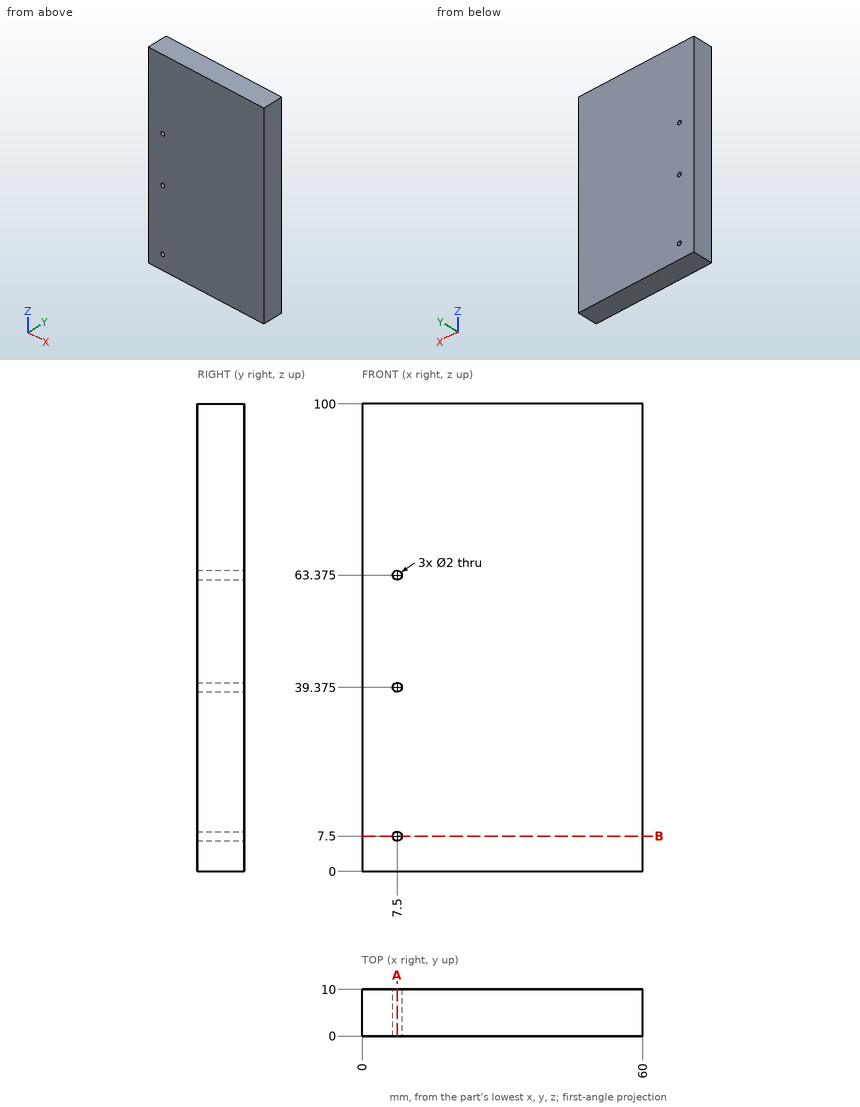
Geometry: see drawing. Coordinates: mm, zero at the bounding-box minimum. Coordinates: 2 decimals unless noted, no trailing zeros. Loops run counter-clockwise (first coordinate to the right, second up) from the corner with the lowest first, then second, coordinate; pieces in that order, holes last. Notation, with made-up numbers: (27, -23.75) -> (77, -23.75) arc R30 ccw to (77, 1.25) -> close; hole circle Ø4 at (0, -3). An arc over 180 degrees is marked (long way). Use a Markdown table: item, result.
1) Cut plane B-B (z = 7.5). Return the cut outline in (x, y), then the cut area to 3 significant figures.
Results found:
| item | result |
|---|---|
| outline | (0, 0) -> (6.5, 0) -> (6.5, 10) -> (0, 10) -> close; (8.5, 0) -> (60, 0) -> (60, 10) -> (8.5, 10) -> close |
| area | 580 mm2 |
2) Material intervals for line 1 along Z through (x, y) = (7.5, 7.5) (3 decimals); line 2 along X through (y, z) = (5.5, 7.5); line 3 along X through (y, z) = (8.5, 38.5), sorted ascending. Write a range as from..to.
Results found:
| item | result |
|---|---|
| line 1 | z = 0..6.5, 8.5..38.375, 40.375..62.375, 64.375..100 |
| line 2 | x = 0..6.5, 8.5..60 |
| line 3 | x = 0..7.02, 7.98..60 |
3) Cut plane A-A (x = 7.5). Return the cut outline in (y, z) (3 decimals), then the cut area to 3 significant figures.
Results found:
| item | result |
|---|---|
| outline | (0, 0) -> (10, 0) -> (10, 6.5) -> (0, 6.5) -> close; (0, 8.5) -> (10, 8.5) -> (10, 38.375) -> (0, 38.375) -> close; (0, 40.375) -> (10, 40.375) -> (10, 62.375) -> (0, 62.375) -> close; (0, 64.375) -> (10, 64.375) -> (10, 100) -> (0, 100) -> close |
| area | 940 mm2 |
